Verification items for the finished model (mm, model axes). Face numbers are marked on the shaded views. A direction names the side the tool comes from. Give positions to 0.01 mm unless a question says otherwise; leave off trailing zeros. Write each loop counter-clockwise with the first axis right and the second up, starting at its lowest first coordinate (ties: lowest second). Pieces come first, ordered by that corner, then holes. Notation, with made-up numbers: (5, 82.25) -> (59, 82.25) arc R9 ccw to (59, 97.25) -> close; hole circle Ø2 at (33, -17.5). An arc over 180 degrees is marked (long way). Answer as CSV lines item,"result". Start each with the question number.
1) Sectioned sample at C-C on y = 4. Record the cut outline in (x, z), and give its area (3 significant figures).
2) Sectioned sample at B-B on x = 2.25. Record the cut outline in (y, z).
3) Sectioned sample at A-A on z = -7.5. Record the cut outline in (x, y).
4) Sectioned sample at D-D on z = 0. Record the cut outline in (x, y).
5) Mould release check, pull along Z, two halves, no side actions. Record for the marked faces 4, 5 and 6: released by +Z, released by -Z, zero draft, split by the parting line, or undercut.
6) Material ranges on L1, parallel to X at y = 4.5, z = 0; L2, parallel to Y at x = 6, z = -4.25; L3, parallel to Y at x = 5.25, z = -2.5, recorded low to high.
7) Gauge pin test, flat ends, axial feed: pin 1 Ø3 at (x, y) = (-1, 4) entering from +Z; pin 2 Ø8 at (x, z) = (0, 0) entering from +Y; pin 3 Ø1.5 at (x, z) = (-5, 6.5) entering from +Y. Record the tip position at first contact, or that the pin passes through.
8) Tool access check on the marked faces 1, 2 and 3. Record the directions out of +Z, -Z, +X, -X, +Y, -Y that give a thin tool (end or side, any length) a straight path to the whole face; none if there is none.
```python
from build123d import *

# Parameters (mm, degrees)
SKETCH1_W               = 21
SKETCH1_H               = 21
BOSS_EXTRUDE1_DEPTH     = 2
BOSS_EXTRUDE2_START     = -2
BOSS_EXTRUDE2_DEPTH     = 2
SKETCH3_R               = 1.6
CUT_EXTRUDE1_DEPTH      = 16.378556499
SKETCH5_R               = 7
BOSS_EXTRUDE3_DEPTH     = 10
SKETCH6_R               = 6.5
CUT_EXTRUDE2_DEPTH      = 10
CUT_EXTRUDE3_REACH      = 25.675
CUT_EXTRUDE3_END_RADIUS = 6.5
BOSS_EXTRUDE4_DEPTH     = 4
SKETCH14_R              = 0.5
CUT_EXTRUDE4_DEPTH      = 10
FILLET1_R               = 4


with BuildPart() as part:
    # Sketch1 → Boss-Extrude1 (new body)
    with BuildSketch(Plane(origin=(0, 0, 0), x_dir=(1, 0, 0), z_dir=(0, 1, 0))):
        Rectangle(SKETCH1_W, SKETCH1_H)
    extrude(amount=BOSS_EXTRUDE1_DEPTH)

    # Sketch4 → Boss-Extrude2 (add)
    with BuildSketch(Plane(origin=(0, 2, 0), x_dir=(1, 0, 0), z_dir=(0, 1, 0)).offset(BOSS_EXTRUDE2_START)):
        with BuildLine():
            Line((-5.761508712, -1.270833333), (-6.632541509, -1.270833333))
            Line((-6.632541509, -1.270833333), (-6.632541509, 1.229166667))
            Line((-6.632541509, 1.229166667), (-5.770541509, 1.229166667))
            ThreePointArc((-5.770541509, 1.229166667), (0, 5.9), (5.770541509, 1.229166667))
            Line((5.770541509, 1.229166667), (6.632541509, 1.229166667))
            Line((6.632541509, 1.229166667), (6.632541509, -1.270833333))
            Line((6.632541509, -1.270833333), (5.761508712, -1.270833333))
            ThreePointArc((5.761508712, -1.270833333), (0, -5.9), (-5.761508712, -1.270833333))
        make_face()
    extrude(amount=-BOSS_EXTRUDE2_DEPTH)

    # Sketch3 → Cut-Extrude1 (cut, through all)
    with BuildSketch(Plane(origin=(0, 2, 0), x_dir=(1, 0, 0), z_dir=(0, 1, 0))):
        with Locations(Location((-7.5, 7.5, 0), (0, 0, 270))):
            Circle(SKETCH3_R)
        with Locations(Location((7.5, 7.5, 0), (0, 0, 270))):
            Circle(SKETCH3_R)
        with Locations(Location((7.5, -7.5, 0), (0, 0, 270))):
            Circle(SKETCH3_R)
        with Locations(Location((-7.5, -7.5, 0), (0, 0, 270))):
            Circle(SKETCH3_R)
    extrude(amount=-CUT_EXTRUDE1_DEPTH, mode=Mode.SUBTRACT)

    # Sketch5 → Boss-Extrude3 (add)
    with BuildSketch(Plane(origin=(0, 2, 0), x_dir=(1, 0, 0), z_dir=(0, 1, 0))):
        with Locations(Location((0, 0, 0), (0, 0, 270))):
            Circle(SKETCH5_R)
    extrude(amount=BOSS_EXTRUDE3_DEPTH)

    # Sketch6 → Cut-Extrude2 (cut)
    with BuildSketch(Plane(origin=(0, 12, 0), x_dir=(1, 0, 0), z_dir=(0, 1, 0))):
        with Locations(Location((0, 0, 0), (0, 0, 270))):
            Circle(SKETCH6_R)
    extrude(amount=-CUT_EXTRUDE2_DEPTH, mode=Mode.SUBTRACT)

    # Cut-Extrude3: up to this cylinder (the profile starts outside it)
    cut_extrude3_end = Plane(origin=(0, 3.932073, 0), z_dir=(0, 1, 0)) * Cylinder(CUT_EXTRUDE3_END_RADIUS, 65.35, mode=Mode.PRIVATE)
    # Sketch12 → Cut-Extrude3 (cut, up to the surface)
    with BuildSketch(Plane.XY.offset(7), mode=Mode.PRIVATE) as cut_extrude3_sk1:
        with BuildLine():
            Line((0.5734508, 2.691842334), (-0.5734508, 2.691842334))
            ThreePointArc((-0.5734508, 2.691842334), (-1.813681206, 3.93207274), (-0.5734508, 5.172303147))
            Line((-0.5734508, 5.172303147), (0.5734508, 5.172303147))
            ThreePointArc((0.5734508, 5.172303147), (1.813681206, 3.93207274), (0.5734508, 2.691842334))
        make_face()
    cut_extrude3_tool1 = extrude(cut_extrude3_sk1.sketch, amount=-CUT_EXTRUDE3_REACH, mode=Mode.PRIVATE) - cut_extrude3_end
    add(cut_extrude3_tool1.solids().sort_by_distance((0, 3.932073, 7))[0], mode=Mode.SUBTRACT)

    # Sketch13 → Boss-Extrude4 (add)
    with BuildSketch(Plane(origin=(0, 2, 0), x_dir=(1, 0, 0), z_dir=(0, 1, 0))):
        Polygon((-2.85, -4.69012427), (2.85, -4.69012427), (3.35, -4.69012427), (3.35, -1.69012427), (2.85, -1.69012427), (2.85, -4.19012427), (-2.85, -4.19012427), (-2.85, -1.69012427), (-3.35, -1.69012427), (-3.35, -4.69012427), align=None)
    extrude(amount=BOSS_EXTRUDE4_DEPTH)

    # Sketch14 → Cut-Extrude4 (cut)
    with BuildSketch(Plane(origin=(0, 0, 4.19012427), x_dir=(-1, 0, 0), z_dir=(0, 0, -1))):
        with Locations((-2.1375, 4)):
            Circle(SKETCH14_R)
        with Locations((-0.7125, 4)):
            Circle(SKETCH14_R)
        with Locations((0.7125, 4)):
            Circle(SKETCH14_R)
        with Locations((2.1375, 4)):
            Circle(SKETCH14_R)
    extrude(amount=-CUT_EXTRUDE4_DEPTH, mode=Mode.SUBTRACT)

    # Fillet1
    fillet1_edges = [part.edges().sort_by_distance(p)[0] for p in [
        (-10.5, 1, -10.5),
        (10.5, 1, -10.5),
        (10.5, 1, 10.5),
        (-10.5, 1, 10.5),
    ]]
    fillet(fillet1_edges, radius=FILLET1_R)


solid = part.part
```
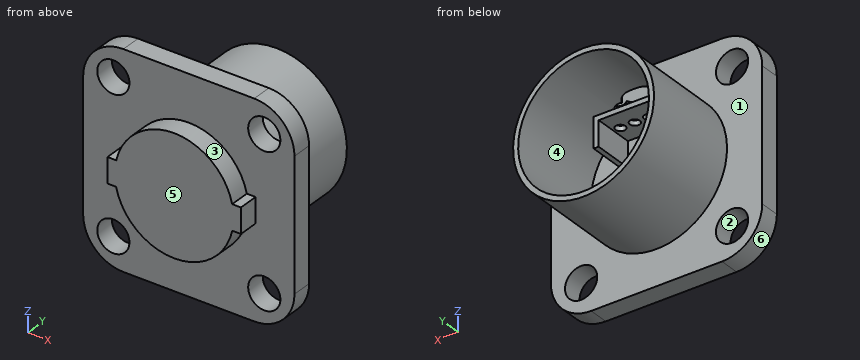
Ans:
1,outline,"(-3.35, 1.69) -> (-2.85, 1.69) -> (-2.85, 4.19) -> (-2.64, 4.19) -> (-2.64, 4.69) -> (-3.35, 4.69) -> close; (-2.64, 5.94) -> (-2.64, 6.48) arc R7 ccw (long way) to (2.64, 6.48) -> (2.64, 5.94) arc R6.5 cw (long way) to start; (-1.64, 4.19) -> (-1.21, 4.19) -> (-1.21, 4.69) -> (-1.64, 4.69) -> close; (-0.21, 4.19) -> (0.21, 4.19) -> (0.21, 4.69) -> (-0.21, 4.69) -> close; (1.21, 4.19) -> (1.64, 4.19) -> (1.64, 4.69) -> (1.21, 4.69) -> close; (2.64, 4.19) -> (2.85, 4.19) -> (2.85, 1.69) -> (3.35, 1.69) -> (3.35, 4.69) -> (2.64, 4.69) -> close"
1,area,"22.3 mm²"
2,outline,"(-2, -5.45) -> (0, -5.45) -> (0, -10.5) -> (2, -10.5) -> (2, -6.63) -> (12, -6.63) -> (12, -6.1) -> (2, -6.1) -> (2, 4.19) -> (3.51, 4.19) -> (3.51, 4.69) -> (2, 4.69) -> (2, 6.1) -> (3.51, 6.1) -> (3.51, 6.63) -> (2, 6.63) -> (2, 10.5) -> (0, 10.5) -> (0, 5.45) -> (-2, 5.45) -> close; (4.49, 4.19) -> (6, 4.19) -> (6, 4.69) -> (4.49, 4.69) -> close; (4.49, 6.1) -> (12, 6.1) -> (12, 6.63) -> (4.49, 6.63) -> close"
3,outline,"(-10.37, 0) -> (-9.1, 0) -> (-9.1, 2) -> (-10.37, 2) -> close; (-5.9, 0) -> (5.9, 0) -> (5.9, 2) -> (-5.9, 2) -> close; (9.1, 0) -> (10.37, 0) -> (10.37, 2) -> (9.1, 2) -> close"
4,outline,"(-10.5, 0) -> (-6.63, 0) -> (-6.63, -2) -> (6.63, -2) -> (6.63, 0) -> (10.5, 0) -> (10.5, 2) -> (7, 2) -> (7, 12) -> (6.5, 12) -> (6.5, 2) -> (-6.5, 2) -> (-6.5, 12) -> (-7, 12) -> (-7, 2) -> (-10.5, 2) -> close"
5,face 4,"undercut"
5,face 5,"zero draft"
5,face 6,"released by -Z"
6,L1,"x = -7 to -6.5, 6.5 to 7"
6,L2,"y = 0 to 2"
6,L3,"y = -2 to 2"
7,pin 1,"stops at z = 7"
7,pin 2,"stops at y = 6"
7,pin 3,"stops at y = 2"
8,face 1,"+Y"
8,face 2,"+Y, -Y"
8,face 3,"+Z, -Y"
